from build123d import *

# Parameters (mm, degrees)
SKETCH1_R           = 16
SKETCH1_R_2         = 1.9
BOSS_EXTRUDE1_DEPTH = 12
SKETCH3_R           = 16
SKETCH3_RX          = 13.630217139
SKETCH3_RY          = 10.086360683
CUT_EXTRUDE2_DEPTH  = 9
REVOLVE1_ANGLE      = 14
CUT_EXTRUDE3_DEPTH  = 9


# Read off the part's stored shape, not the designer's step: Revolve1
with BuildPart() as part:
    # Sketch1 → Boss-Extrude1 (new body)
    with BuildSketch(Plane(origin=(0, 0, 0), x_dir=(1, 0, 0), z_dir=(0, 1, 0))):
        with Locations(Location((0, 0, 0), (0, 0, 270))):
            Circle(SKETCH1_R)
        with Locations(Location((-9.95, 0, 0), (0, 0, 270))):
            Circle(SKETCH1_R_2, mode=Mode.SUBTRACT)
        with Locations(Location((9.95, 0, 0), (0, 0, 270))):
            Circle(SKETCH1_R_2, mode=Mode.SUBTRACT)
        with Locations(Location((0, 0, 0), (0, 0, 270))):
            Circle(SKETCH1_R_2, mode=Mode.SUBTRACT)
    extrude(amount=BOSS_EXTRUDE1_DEPTH)

    # Sketch3 → Cut-Extrude2 (cut)
    with BuildSketch(Plane.XZ):
        with Locations(Location((0, 0, 0), (0, 0, 90))):
            Circle(SKETCH3_R)
        with Locations(Location((0, 0), (0, 0, 180))):
            Ellipse(SKETCH3_RX, SKETCH3_RY, mode=Mode.SUBTRACT)
    extrude(amount=-CUT_EXTRUDE2_DEPTH, mode=Mode.SUBTRACT)

    # Revolve1 outline → Revolve1 (revolve)
    with BuildSketch(Plane(origin=(0, 0, 0), x_dir=(-0.12186934340514781, 0, 0.992546151641322), z_dir=(-0.992546151641322, 0, -0.12186934340514781))):
        Polygon((10.086360682, 9), (10.086360682, -1e-09), (16, 9), align=None)
    revolve1 = revolve(axis=Axis((0, 0, 0), (0, 1, 0)), revolution_arc=REVOLVE1_ANGLE)

    # Mirror1: Revolve1 across plane
    add(revolve1.mirror(Plane.XY))

    # Sketch6 → Cut-Extrude3 (cut)
    with BuildSketch(Plane.XZ):
        Polygon((3.464101615, 6), (-3.464101615, 6), (-6.92820323, 0), (-3.464101615, -6), (3.464101615, -6), (6.92820323, 0), align=None)
    extrude(amount=-CUT_EXTRUDE3_DEPTH, mode=Mode.SUBTRACT)


solid = part.part
For this review, take the finished solid that the model builds, in its own axes (mm). A direction names the side the tool comes from. Round coordinates to 2 decimals unless told otherwise and drop trailing zeros. Write each loop counter-clockwise with the first axis right and the second up, starting at its lowest first coordinate (ties: lowest second). Pieces come first, ordered by that corner, then holes. Notation, with made-up numbers: (29.25, 6.5) -> (69.25, 6.5) arc R28 cw to (69.25, 44.5) -> close; hole circle Ø10 at (-30.5, 84.25). An arc over 180 degrees is marked (long way). Put each result on its own line as item: value.
Q1. The part is to be moulded in two halves that separate along X. For faces 1 (the flat face through (1.507, 5.583, -12.274)), 2 (the flat face through (-1.507, 5.583, 12.274)), 3 (the flat face through (0, 4, 6)), say which applies: released by +X, released by -X, zero draft, split by the parting line, or undercut.
Determined:
face 1: released by +X
face 2: released by -X
face 3: undercut
Q2. Machinability: for faces 4 (the flat face through (13.4, 9, 3.3)), 5 (the flat face through (0, 4, -6)), 6 (the flat face through (-1.507, 5.583, -12.274)), which of the approach directions +Z, -Z, +X, -X, +Y, -Y give a long, thin tool a straight path to every point of the face, cutting with its end or side? Answer none if there is none.
Determined:
face 4: +X, -Y
face 5: -Y
face 6: -X, -Y
Q3. Consider section B-B on z = 1. Give the number of separate pieces and of enclosed holes in the cut face, and give its area (3 significant figures).
Determined:
separate pieces: 4
enclosed holes: 0
area: 138 mm^2
Q4. To check wall thickness, follow L1, parallel to X at y = 10.15, z = 0; L2, parallel to X at y = 7.75, z = 1.5; L3, parallel to Y at x = 0, z = 3.5. State the ranges of each line that lie inside material, in increasing order. Write a range as [from, to].
Determined:
L1: x = [-16, -11.85], [-8.05, -1.9], [1.9, 8.05], [11.85, 16]
L2: x = [-13.48, -11.12], [-8.78, -6.06], [6.06, 8.78], [11.12, 13.48]
L3: y = [9, 12]
Q5. Clearance check with flat-ended pins moving along their axes: pin 1 Ø2 at (y, z) = (1.5, 5.5) entering from -X; pin 2 Ø5.5 at (x, y) = (-1.5, 6.5) entering from +Z; pin 3 Ø3 at (x, y) = (10, 8.5) entering from +Z. State where each tip first meets the part, or that it passes through.
Determined:
pin 1: stops at x = -12.2
pin 2: stops at z = 16
pin 3: stops at z = 13.5
Q6. Consider section A-A on y = 11. State the section outline as (x, z) points.
Determined:
outline: circle Ø32 at (0, 0); hole circle Ø3.8 at (-9.95, 0); hole circle Ø3.8 at (0, 0); hole circle Ø3.8 at (9.95, 0)
